```python
from build123d import *

# Parameters (mm, degrees)
SKETCH1_W           = 130
SKETCH1_H           = 80
BOSS_EXTRUDE1_DEPTH = 2.5
SKETCH2_W           = 110
SKETCH2_H           = 60
CUT_EXTRUDE1_DEPTH  = 1.25
SKETCH3_R           = 1.5
CUT_EXTRUDE2_DEPTH  = 153.663846408
SKETCH4_W           = 50
SKETCH4_H           = 30
CUT_EXTRUDE3_DEPTH  = 153.648493278


with BuildPart() as part:
    # Sketch1 → Boss-Extrude1 (new body)
    with BuildSketch(Plane(origin=(0, 0, 0), x_dir=(1, 0, 0), z_dir=(0, 1, 0))):
        with Locations((65, 40)):
            Rectangle(SKETCH1_W, SKETCH1_H)
    extrude(amount=BOSS_EXTRUDE1_DEPTH)

    # Sketch2 → Cut-Extrude1 (cut)
    with BuildSketch(Plane(origin=(0, 2.5, 0), x_dir=(1, 0, 0), z_dir=(0, 1, 0))):
        with Locations((65, 40)):
            Rectangle(SKETCH2_W, SKETCH2_H)
    extrude(amount=-CUT_EXTRUDE1_DEPTH, mode=Mode.SUBTRACT)

    # Sketch3 → Cut-Extrude2 (cut, through all)
    with BuildSketch(Plane(origin=(0, 2.5, 0), x_dir=(1, 0, 0), z_dir=(0, 1, 0))):
        with Locations(Location((5, 75, 0), (0, 0, 270))):
            Circle(SKETCH3_R)
        with Locations(Location((125, 75, 0), (0, 0, 270))):
            Circle(SKETCH3_R)
        with Locations(Location((125, 5, 0), (0, 0, 270))):
            Circle(SKETCH3_R)
        with Locations(Location((5, 5, 0), (0, 0, 270))):
            Circle(SKETCH3_R)
    extrude(amount=-CUT_EXTRUDE2_DEPTH, mode=Mode.SUBTRACT)

    # Sketch4 → Cut-Extrude3 (cut, through all)
    with BuildSketch(Plane(origin=(0, 1.25, 0), x_dir=(1, 0, 0), z_dir=(0, 1, 0))):
        with Locations((65, 40)):
            Rectangle(SKETCH4_W, SKETCH4_H)
    extrude(amount=-CUT_EXTRUDE3_DEPTH, mode=Mode.SUBTRACT)


solid = part.part
```
Check sheet for the modelled part. Datum: model origin and axes. Units: mm. Give positions to 0.01 mm unless a question says otherwise; leave off trailing zeros. Order: outer loops, then holes, each group sorted by start corner. A loop starts at its lowest first (then second) coordinate and runs counter-clockwise, first axis right, second up. Notation, with made-up numbers: M 51.5,66 L 73.5,66 A19 ccw 73.5,97 Z; hole C -6.75,-1 d7. An arc over 180 degrees is marked long. Answer in a Markdown table with one row per item.
1) Cross-section at A-A, the plane z = -75. Enter the section's corners in (x, y), plus the area to 3 significant figures.
Filled sheet:
| item | result |
|---|---|
| outline | M 0,0 L 3.5,0 L 3.5,2.5 L 0,2.5 Z; M 6.5,0 L 123.5,0 L 123.5,2.5 L 6.5,2.5 Z; M 126.5,0 L 130,0 L 130,2.5 L 126.5,2.5 Z |
| area | 310 mm2 |
2) Cross-section at C-C, the plane x = 125. Enter the section's corners in (y, z).
Filled sheet:
| item | result |
|---|---|
| outline | M 0,-80 L 2.5,-80 L 2.5,-76.5 L 0,-76.5 Z; M 0,-73.5 L 2.5,-73.5 L 2.5,-6.5 L 0,-6.5 Z; M 0,-3.5 L 2.5,-3.5 L 2.5,0 L 0,0 Z |
3) Release check for a two-part mould opening along Z. For faces 1 (the flat face through (64, 1.25, -60)), 2 (the cylindrical face through (5.45, 1.27, -73.57)), 3 (the flat face through (64, 1, 0)), 4 (the flat face through (130, 1, -39)) record: +Z half, -Z half, draft (parallel to the pull), parting line (faces both ways), or undercut.
Filled sheet:
| item | result |
|---|---|
| face 1 | undercut |
| face 2 | undercut |
| face 3 | +Z half |
| face 4 | draft |
4) Gauge pin test, flat end, axial feed: P1, Ø6, axis at x = 67.5, z = -26, coming from the +Y side. Record the tip position at first contact, or that the pin passes through.
Filled sheet:
| item | result |
|---|---|
| P1 | stops at y = 1.25 |
5) Cross-section at D-D, the plane z = -27. Enter the section's corners in (x, y).
Filled sheet:
| item | result |
|---|---|
| outline | M 0,0 L 40,0 L 40,1.25 L 10,1.25 L 10,2.5 L 0,2.5 Z; M 90,0 L 130,0 L 130,2.5 L 120,2.5 L 120,1.25 L 90,1.25 Z |
6) Thickness scan on L1, parallel to X at y = 1.75, z = -5; L2, parallel to Z at x = 125, y = 1.65; L3, parallel to Z at x = 86.5, y = 1.95. Record the ranges inside material, lowest first. Write a range as [from, to].
Filled sheet:
| item | result |
|---|---|
| L1 | x = [0, 3.5], [6.5, 123.5], [126.5, 130] |
| L2 | z = [-80, -76.5], [-73.5, -6.5], [-3.5, 0] |
| L3 | z = [-80, -70], [-10, 0] |
7) Cross-section at B-B, the plane y = 2.1. Enter the section's corners in (x, z).
Filled sheet:
| item | result |
|---|---|
| outline | M 0,-80 L 130,-80 L 130,0 L 0,0 Z; hole C 5,-75 d3; hole C 5,-5 d3; hole M 10,-70 L 120,-70 L 120,-10 L 10,-10 Z; hole C 125,-75 d3; hole C 125,-5 d3 |
